For this review, take the finished solid that the model builds, in its own axes (mm). A direction names the side the tool comes from. Give positions to 0.01 mm unless a question says otherwise; leave off trailing zeros. Loops run counter-clockwise (first coordinate to the right, second up) from the corner with the lowest first, then second, coordinate; pieces in that order, holes last. Notation, with made-up numbers: (19, -18.75) - (58, -18.75) arc R8 ccw to (58, -12.75) - close; hole circle Ø1 at (-10.5, 23). An arc over 180 degrees is marked (long way). Answer in a Markdown table with one row per item.
```python
from build123d import *

# Parameters (mm, degrees)
BOSS_EXTRUDE1_DEPTH            = 10
CBORE_FOR_M5_SHCS1_AT_2_COUNT  = 2
CBORE_FOR_M5_SHCS1_AT_2_PITCH  = 20
FILLET1_R                      = 2
CUT_EXTRUDE1_DEPTH             = 4.2
M5_CLEARANCE_HOLE1_D           = 5.5
M5_CLEARANCE_HOLE1_CSINK_D     = 5.55
M5_CLEARANCE_HOLE1_CSINK_ANGLE = 90
SKETCH9_R                      = 10
SKETCH9_R_2                    = 2.75
BOSS_EXTRUDE2_DEPTH            = 7.9


with BuildPart() as part:
    # Sketch1 → Boss-Extrude1 (new body)
    with BuildSketch(Plane(origin=(0, 0, 0), x_dir=(1, 0, 0), z_dir=(0, 1, 0))):
        Polygon((0, 0), (40, 0), (40, 43.75), (20, 43.75), (20, 20), (0, 20), align=None)
    extrude(amount=BOSS_EXTRUDE1_DEPTH)

    # Sketch4 → CBORE for M5 SHCS1 (revolve, cut)
    with BuildSketch(Plane(origin=(10, 0, -10), x_dir=(0, 0, -1), z_dir=(1, 0, 0))):
        Polygon((0, 0), (0, 10), (2.75, 10), (2.75, 5), (5, 5), (5, 0.025), (5.025, 0), align=None)
    cbore_for_m5_shcs1 = revolve(axis=Axis((10, -6.35, -10), (0, 1, 0)), mode=Mode.SUBTRACT)

    # CBORE for M5 SHCS1 at 2: CBORE for M5 SHCS1 ×2
    with Locations(*[(i * CBORE_FOR_M5_SHCS1_AT_2_PITCH, 0, 0) for i in range(1, CBORE_FOR_M5_SHCS1_AT_2_COUNT)]):
        add(cbore_for_m5_shcs1, mode=Mode.SUBTRACT)

    # Fillet1
    fillet1_edges = [part.edges().sort_by_distance(p)[0] for p in [
        (0, 5, -20),
        (20, 5, -20),
        (20, 5, -43.75),
        (40, 5, -43.75),
        (40, 5, 0),
        (0, 5, 0),
    ]]
    fillet(fillet1_edges, radius=FILLET1_R)

    # Sketch6 → Cut-Extrude1 (cut)
    with BuildSketch(Plane.XZ):
        Polygon((34.7, -33.75), (32.35, -29.679680602), (27.65, -29.679680602), (25.3, -33.75), (27.65, -37.820319398), (32.35, -37.820319398), align=None)
    extrude(amount=-CUT_EXTRUDE1_DEPTH, mode=Mode.SUBTRACT)

    # M5 Clearance Hole1 (through all)
    with Locations(Plane(origin=(0, 0, 0), x_dir=(-1, 0, 0), z_dir=(0, -1, 0))):
        with Locations((-30, 33.75)):
            CounterSinkHole(M5_CLEARANCE_HOLE1_D / 2, M5_CLEARANCE_HOLE1_CSINK_D / 2, counter_sink_angle=M5_CLEARANCE_HOLE1_CSINK_ANGLE)

    # Sketch9 → Boss-Extrude2 (add)
    with BuildSketch(Plane(origin=(0, 10, 0), x_dir=(1, 0, 0), z_dir=(0, 1, 0))):
        with Locations((30, 33.75)):
            Circle(SKETCH9_R)
        with Locations((30, 33.75)):
            Circle(SKETCH9_R_2, mode=Mode.SUBTRACT)
    extrude(amount=BOSS_EXTRUDE2_DEPTH)


solid = part.part
```
1. For faces 4 (the face through (22, 10, -42)), 5 (the face through (24, 0, -17)), 6 (the face through (30, 2, -37.82)), 7 (the face through (34.614, 13.895, -24.878)), list the 3-axis set-ups (+Z, -Z, +X, -X, +Y, -Y) from which the entire face can be reached by the end or side of a thin tool; tool diameter is ignored.
Values:
| item | result |
|---|---|
| face 4 | -Z, -X, +Y |
| face 5 | +Z, -Z, +X, -X, -Y |
| face 6 | -Y |
| face 7 | +Y |
2. We need section A-A, the plane z = -10. Give the boundary of the cut face in (x, y) (3 decimals).
Values:
| item | result |
|---|---|
| outline | (0, 0) - (4.975, 0) - (5, 0.025) - (5, 5) - (7.25, 5) - (7.25, 10) - (0, 10) - close; (12.75, 5) - (15, 5) - (15, 0.025) - (15.025, 0) - (24.975, 0) - (25, 0.025) - (25, 5) - (27.25, 5) - (27.25, 10) - (12.75, 10) - close; (32.75, 5) - (35, 5) - (35, 0.025) - (35.025, 0) - (40, 0) - (40, 10) - (32.75, 10) - close |
3. Clearance check with flat-ended pins moving along their axes: pin 1 (1 mm diameter, centred on x = 11, y = 5.5, fed in from -Z); pin 2 (11.5 mm diameter, centred on x = 30, z = -10, fed in from -Y); pin 3 (3 mm diameter, centred on y = 5.5, z = -34.5, fed in from -X); pin 4 (5 mm diameter, centred on x = 30, z = -11, fed in from -Y). State where each tip first meets the part, or that it passes through.
Values:
| item | result |
|---|---|
| pin 1 | stops at z = -20 |
| pin 2 | stops at y = 0 |
| pin 3 | stops at x = 20 |
| pin 4 | stops at y = 5 |
4. We need section C-C, the plane y = 10.5. Give the boundary of the cut face in (x, z).
Values:
| item | result |
|---|---|
| outline | circle Ø20 at (30, -33.75); hole circle Ø5.5 at (30, -33.75) |
5. Wall thickness on line 1 (Z direction, x = 30, y = 8.25); line 2 (X direction, y = 2, z = -10); line 3 (Z direction, x = 30, y = 1.6): over which ranges is each line inside the solid? List them lowest first. Write a range as [from, to].
Values:
| item | result |
|---|---|
| line 1 | z = [-43.75, -36.5], [-31, -12.75], [-7.25, 0] |
| line 2 | x = [0, 5], [15, 25], [35, 40] |
| line 3 | z = [-43.75, -37.82], [-29.68, -15], [-5, 0] |
6. We need section B-B, the plane z = -32.5. Give the boundary of the cut face in (x, y).
Values:
| item | result |
|---|---|
| outline | (20, 0) - (26.02, 0) - (26.02, 4.2) - (27.55, 4.2) - (27.55, 17.9) - (20.08, 17.9) - (20.08, 10) - (20, 10) - close; (32.45, 4.2) - (33.98, 4.2) - (33.98, 0) - (40, 0) - (40, 10) - (39.92, 10) - (39.92, 17.9) - (32.45, 17.9) - close |
7. Mouldability with a two-part tool opening along X and no side actions: class faces 1 (the face through (20, 10, -10)), 2 (the face through (20, 5, -32)), 3 (the face through (33.54, 2.07, -31.74)) as released by +X, released by -X, zero draft, split by the parting line, or undercut.
Values:
| item | result |
|---|---|
| face 1 | zero draft |
| face 2 | released by -X |
| face 3 | undercut |
8. We need section D-D, the plane x = 21. Give the boundary of the cut face in (y, z).
Values:
| item | result |
|---|---|
| outline | (0, -43.48) - (10, -43.48) - (10, -38.11) - (17.9, -38.11) - (17.9, -29.39) - (10, -29.39) - (10, 0) - (0, 0) - close |
